Can you work these out from the drawing? Everything is in mm from the part's minimum corner. Give positions to 0.01 mm unless a question says otherwise; leave off trailing zeros. Order: outer loops, then holes, each group sorted by start corner. A loop starts at its lowest first (then second) coordinate and runs counter-clockwise, first axis right, second up. Notation, with made-up numbers: (-18.75, 44.5) -> (9.25, 44.5) arc R29 cw to (9.25, 69.5) -> close; hole circle Ø3 at (35.25, -35). An arc over 180 degrees is marked (long way). One line per item, written item: value.
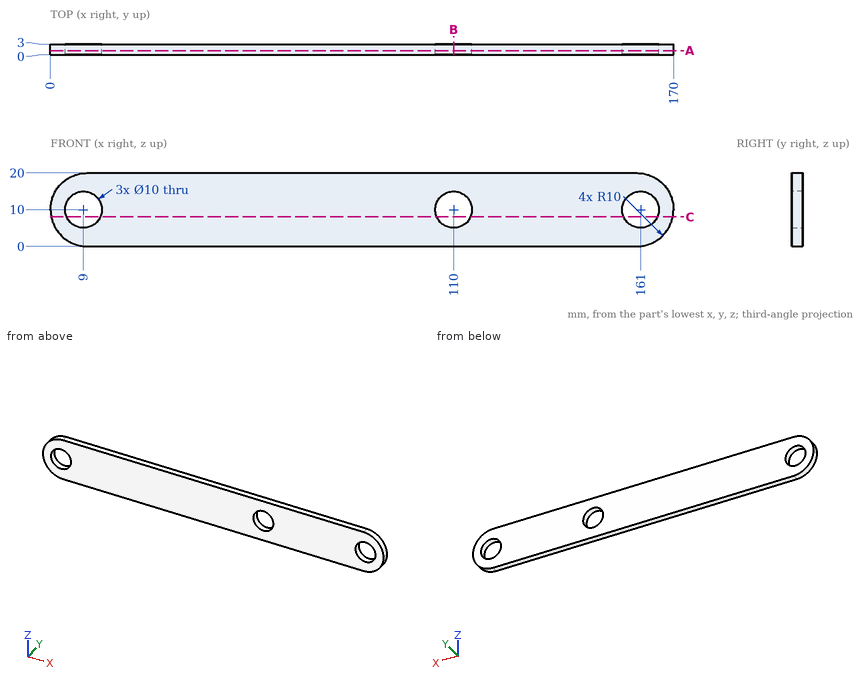
1) Suppose I cut it at B-B, the plane x = 110. Write out the boundary of the cut face in (y, z), then the cut area to 3 significant figures.
Answer below:
outline: (0, 0) -> (3, 0) -> (3, 5) -> (0, 5) -> close; (0, 15) -> (3, 15) -> (3, 20) -> (0, 20) -> close
area: 30.0 mm2
2) For P1, Ø1.5, axis at y = 2, z = 6, coming from the +X side, with a flat end and sliding along its axis, tell me the tip position at first contact or that it passes through.
Answer below:
P1: stops at x = 169.46
3) Suppose I cut it at A-A, the plane y = 1.2. State how many separate pieces and enclosed holes the cut face has, then the cut area to 3 significant figures.
Answer below:
separate pieces: 1
enclosed holes: 3
area: 3,080 mm2
4) If I drill on line 1 along X through (y, z) = (2.05, 10); line 2 along X through (y, z) = (1.7, 13.25); line 3 along Z through (x, y) = (114, 1.4), over which ranges is the centre line in solid material (lowest first)?
Answer below:
line 1: x = 0 to 4, 14 to 105, 115 to 156, 166 to 170
line 2: x = 0.54 to 5.2, 12.8 to 106.2, 113.8 to 157.2, 164.8 to 169.46
line 3: z = 0 to 7, 13 to 20
5) Suppose I cut it at C-C, the plane z = 8. Write out the boundary of the cut face in (x, y).
Answer below:
outline: (0.2, 0) -> (4.42, 0) -> (4.42, 3) -> (0.2, 3) -> close; (13.58, 0) -> (105.42, 0) -> (105.42, 3) -> (13.58, 3) -> close; (114.58, 0) -> (156.42, 0) -> (156.42, 3) -> (114.58, 3) -> close; (165.58, 0) -> (169.8, 0) -> (169.8, 3) -> (165.58, 3) -> close
